Job drawing, mm, ordinate dimensions from the low corner. One solid piece. Give positions to 0.01 mm unless a question says otherwise; leave off trailing zeros. Order: outer loops, then holes, each group sorted by start corner. A loop starts at its lowest first (then second) coordinate and runs counter-clockwise, first axis right, second up. Notation, with made-up numbers: (0.25, 15) - (34.25, 15) arc R32 ccw to (34.25, 53) - close; hole circle Ø11 at (-18, 88.25). An arc over 180 degrees is marked (long way). Use one line per item in the form item = value. Start each with the question number.
1. Band-saw the part on C-C, the plane z = 83.15. List the corners of the cut face in (x, y).
2. Band-saw the part on A-A, the plane x = 186.6. List the corners of the cut face in (y, z), plus the area to 3 significant figures.
3. Drill centre lines: line 1 (Z direction, x = 169, y = 7.25); line 2 (Z direction, x = 186.6, y = 4); line 3 (X direction, y = 6.5, z = 83.15). Where is each one in solid material? Low to high.
4. Pull direction X, two halves, no side cores. Call the marked faces 1 and 2: +X half, -X half, draft (parallel to the pull), parting line (faces both ways), or undercut.
5. Band-saw the part on B-B, the plane z = 26.5. List the corners of the cut face in (x, y).
6. Pin check, flat tips, straight feed: P1, Ø1.5, axis at y = 3, z = 100, coming from the -X side; P2, Ø2, axis at x = 189.5, z = 89, coming from the -Y side; P3, Ø8, axis at x = 92, z = 67.5, coming from the +Y side; P4, Ø1.5, axis at x = 74.5, y = 8.5, coming from the -Z side. Stop position of each tip, or through.
7. Band-saw the part on D-D, the plane x = 92.5. List the corners of the cut face in (y, z), plus the area to 3 significant figures.
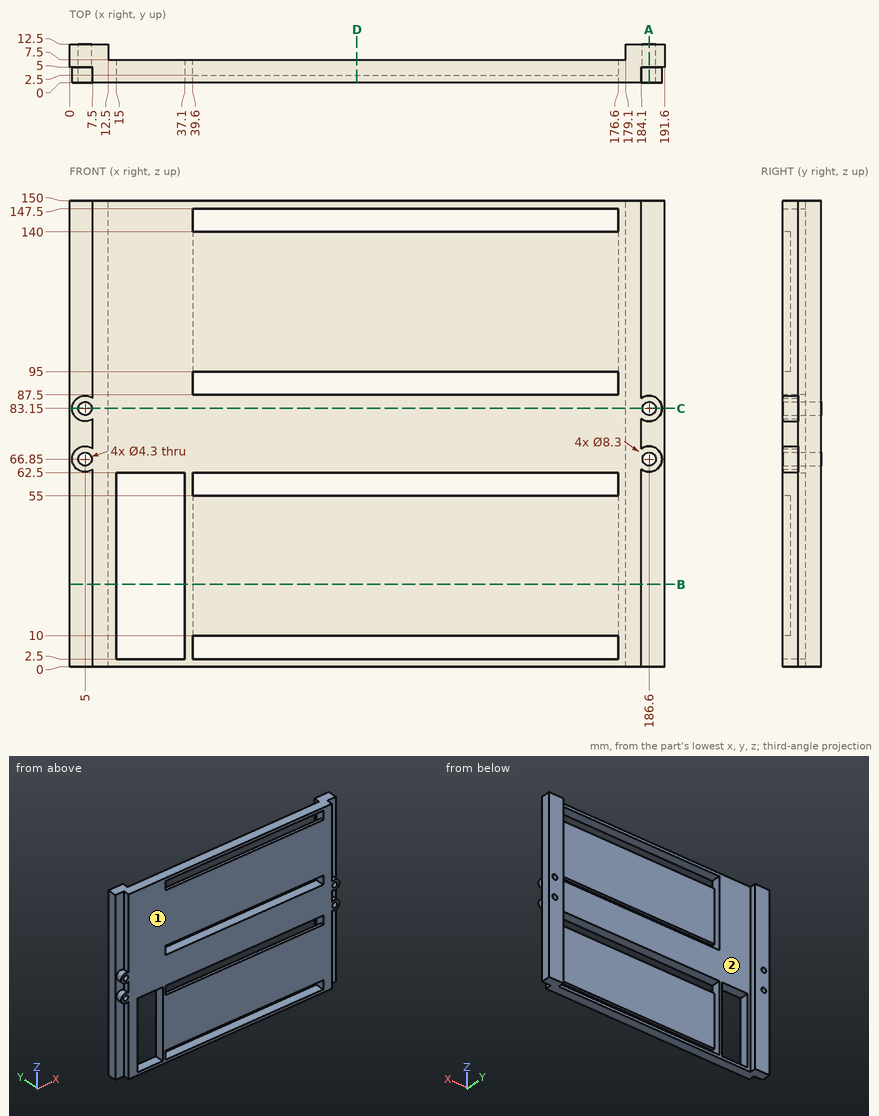
From the geometry:
q1.outline = (0, 5) - (0.85, 5) - (0.85, 0) - (2.85, 0) - (2.85, 12.5) - (0, 12.5) - close; (7.15, 0) - (184.45, 0) - (184.45, 12.5) - (179.1, 12.5) - (179.1, 7.5) - (12.5, 7.5) - (12.5, 12.5) - (7.15, 12.5) - close; (188.75, 0) - (190.75, 0) - (190.75, 5) - (191.6, 5) - (191.6, 12.5) - (188.75, 12.5) - close
q2.outline = (0, 62.7) - (5, 62.7) - (5, 0) - (12.5, 0) - (12.5, 64.7) - (0, 64.7) - close; (0, 69) - (12.5, 69) - (12.5, 81) - (0, 81) - (0, 79) - (5, 79) - (5, 71) - (0, 71) - close; (0, 85.3) - (12.5, 85.3) - (12.5, 150) - (5, 150) - (5, 87.3) - (0, 87.3) - close
q2.area = 1,100 mm²
q3.line_1 = 0 to 2.5, 62.5 to 87.5, 147.5 to 150
q3.line_2 = 62.7 to 64.7, 69 to 71, 79 to 81, 85.3 to 87.3
q3.line_3 = 0 to 2.85, 7.15 to 184.45, 188.75 to 191.6
q4.face_1 = draft
q4.face_2 = undercut
q5.outline = (0, 5) - (7.5, 5) - (7.5, 0) - (15, 0) - (15, 7.5) - (12.5, 7.5) - (12.5, 12.5) - (0, 12.5) - close; (37.1, 0) - (184.1, 0) - (184.1, 5) - (191.6, 5) - (191.6, 12.5) - (179.1, 12.5) - (179.1, 7.5) - (176.6, 7.5) - (176.6, 2.5) - (39.6, 2.5) - (39.6, 7.5) - (37.1, 7.5) - close
q6.P1 = 7.5
q6.P2 = 5
q6.P3 = 7.5
q6.P4 = through
q7.outline = (0, 0) - (7.5, 0) - (7.5, 2.5) - (0, 2.5) - close; (0, 10) - (2.5, 10) - (2.5, 55) - (0, 55) - close; (0, 62.5) - (7.5, 62.5) - (7.5, 87.5) - (0, 87.5) - close; (0, 95) - (2.5, 95) - (2.5, 140) - (0, 140) - close; (0, 147.5) - (7.5, 147.5) - (7.5, 150) - (0, 150) - close
q7.area = 450 mm²
